Could you check a few things on this model? Use its own coordinates, in mm. A direction names the side the tool comes from. Give positions to 0.01 mm unless a question says otherwise; leave off trailing zeros. Write each loop counter-clockwise with the first axis right and the second up, starting at its lowest first coordinate (ties: lowest second). Pieces come first, ordered by that corner, then holes. Notation, with made-up numbers: M -5.75,-27 L 37.25,-27 A18 ccw 37.25,-8 Z; hole C 35,51.5 d6. An arc over 180 degrees is marked long. One line per item, written item: value.
```python
from build123d import *

# Parameters (mm, degrees)
F0_R     = 14.75
F1_DEPTH = 5
F2_R     = 17.375
F3_DEPTH = 9
F5_DEPTH = 15.875
F6_R     = 12
F7_DEPTH = 15
F8_R     = 15.5
F9_DEPTH = 3


# Not quite as in the source:
# - a fillet or chamfer that OpenCascade refuses, or shapes differently, is made with other operations: its cross-section is extruded or revolved along the edge and cut away or added


with BuildPart() as f1:
    # F0 (on Top) → F1 (new body)
    with BuildSketch(Plane.XY):
        Circle(F0_R)
    extrude(amount=F1_DEPTH)

    # F2 (on face) → F3 (join)
    with BuildSketch(Plane.XY.offset(5)):
        Circle(F2_R)
    extrude(amount=F3_DEPTH)

    # F4 (on Right) → F5 (join, symmetric)
    with BuildSketch(Plane.YZ):
        with BuildLine():
            Line((0.5, 3), (-0.5, 3))
            ThreePointArc((-0.5, 3), (-1, 2.5), (-0.5, 2))
            Line((-0.5, 2), (0.5, 2))
            ThreePointArc((0.5, 2), (1, 2.5), (0.5, 3))
        make_face()
    extrude(amount=F5_DEPTH, both=True)

    # F6 (on face) → F7 (cut)
    with BuildSketch(Plane(origin=(0, 0, 0), x_dir=(1, 0, 0), z_dir=(0, 0, -1))):
        Circle(F6_R)
    extrude(amount=-F7_DEPTH, mode=Mode.SUBTRACT)

    # F8 (on face) → F9 (cut)
    with BuildSketch(Plane.XY.offset(14)):
        Circle(F8_R)
    extrude(amount=-F9_DEPTH, mode=Mode.SUBTRACT)

    # F10: fillet of radius 5 on 1 edges, made by hand

    # F10_s1 → F10_t2 (revolve, cut)
    with BuildSketch(Plane.XZ):
        with BuildLine():
            ThreePointArc((17.375, 10.096876251), (16.8819390943, 12.2619397605), (15.5, 14))
            Line((15.5, 14), (17.375, 14))
            Line((17.375, 14), (17.375, 10.096876251))
        make_face()
    revolve(axis=Axis((0, 0, 14), (0, 0, 1)), mode=Mode.SUBTRACT)


solid = f1.part
```
1) If we section it at A-A, the plane x = 0: Write out the boundary of the cut face in (y, z) (3 decimals), then the cut area to 3 significant figures.
Outcome:
outline: M -17.375,5 L -14.75,5 L -14.75,0 L -12,0 L -12,11 L -15.5,11 L -15.5,14 A5 ccw -17.375,10.097 Z; M 12,0 L 14.75,0 L 14.75,5 L 17.375,5 L 17.375,10.097 A5 ccw 15.5,14 L 15.5,11 L 12,11 Z
area: 98.8 mm^2
2) We'd pull the mould along Y, two halves only. Please class faces 1 (the face through (-2.018, 15.368, 12.521)), 2 (the face through (4.5, -11.4, 11)), 3 (the face through (-15, 0, 3)), 4 (the face through (-15.3, 1, 2.5)): pulls with the +Y half, pulls with the -Y half, needs draft (parallel to the pull), parting line crosses it, or undercut.
Outcome:
face 1: undercut
face 2: undercut
face 3: needs draft
face 4: pulls with the +Y half
3) If we section it at D-D, the plane z = 13.25: Write out the boundary of the cut face in (x, y).
Outcome:
outline: C 0,0 d32.51; hole C 0,0 d31
4) I'm going to push flat-ended pins straight in: pin 1 (1.1 mm diameter, centred on x = 15, y = 0, fed in from -Z); pin 2 (4 mm diameter, centred on y = 5.5, z = 3.5, fed in from -X); pin 3 (1 mm diameter, centred on x = -3.5, z = 3, fed in from -Y); pin 4 (0.8 mm diameter, centred on y = 0, z = 2.5, fed in from +X) (3 decimals). Where does each tip first touch, or does it pass through?
Outcome:
pin 1: stops at z = 0
pin 2: stops at x = -16.87
pin 3: stops at y = -14.44
pin 4: stops at x = 15.875
5) Please list where these lines run through material, in increasing order: L1, parallel to Y at x = 0, z = 6 (3 decimals); L2, parallel to Y at x = 0, z = 3; L3, parallel to Z at x = 10, y = 11. Write a range as from..to.
Outcome:
L1: y = -17.375..-12, 12..17.375
L2: y = -14.75..-12, 12..14.75
L3: z = 5..11
6) If we section it at C-C, the plane z = 8: Write out the boundary of the cut face in (x, y) (3 decimals).
Outcome:
outline: C 0,0 d34.75; hole C 0,0 d24
7) If we section it at B-B, the plane z = 2.5: Write out the boundary of the cut face in (x, y) (3 decimals).
Outcome:
outline: M -15.875,-1 L -14.716,-1 A14.75 ccw 14.716,-1 L 15.875,-1 L 15.875,1 L 14.716,1 A14.75 ccw -14.716,1 L -15.875,1 Z; hole C 0,0 d24
8) On a 3-axis mill with a long thin cutter (end or side, diameter ignored), from which of +Z, -Z, +X, -X, +Y, -Y can I reach the whole of each face in a straight line? I mean faces 5 (the face through (15.3, -1, 2.5)), 6 (the face through (-15.875, 0, 2.5)), 7 (the face through (15.3, 1, 2.5)), 8 (the face through (15.875, 0, 2.5)), 9 (the face through (-15.3, -1, 2.5)). Say none if no direction works.
Outcome:
face 5: +X, -Y
face 6: -Z, -X, +Y, -Y
face 7: +X, +Y
face 8: -Z, +X, +Y, -Y
face 9: -X, -Y
